Source: three-view drawing plus pictorial views. Frame: mm from the lowest corner of the part. Round coordinates to 2 decimals unless told otherwise and drop trailing zeros. Write each loop counter-clockwise with the first axis right and the second up, starting at its lowest first coordinate (ties: lowest second). Pieces come first, ordered by that corner, then holes.
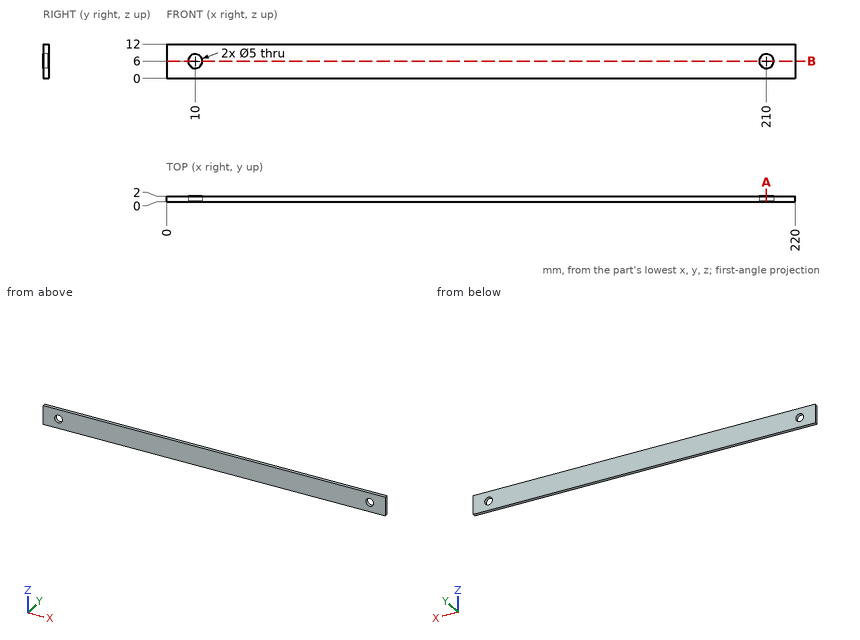
1) Section B-B on z = 6. Output: boundary loops of the cut face in (x, y).
2) Line query: probe 1 along Z at (x, y) = (10, 0.9); probe 2 along X at (y, z) = (1.3, 4); probe 3 along X at (y, z) = (0.9, 5). Output: solid intervals per line, ascending.
3) Section A-A on x = 210. Output: boundary loops of the cut face in (y, z).
Filled in:
1. outline: (0, 0) - (7.5, 0) - (7.5, 2) - (0, 2) - close; (12.5, 0) - (207.5, 0) - (207.5, 2) - (12.5, 2) - close; (212.5, 0) - (220, 0) - (220, 2) - (212.5, 2) - close
2. probe 1: z = 0 to 3.5, 8.5 to 12
2. probe 2: x = 0 to 8.5, 11.5 to 208.5, 211.5 to 220
2. probe 3: x = 0 to 7.71, 12.29 to 207.71, 212.29 to 220
3. outline: (0, 0) - (2, 0) - (2, 3.5) - (0, 3.5) - close; (0, 8.5) - (2, 8.5) - (2, 12) - (0, 12) - close
